Can you work these out from the model? Positions are in its coordinate system, mm. A direction names the side the tool comes from. Give positions to 0.01 mm unless a question says otherwise; leave off trailing zeros. Order: outer loops, then holes, each group sorted by start corner. A loop starts at its lowest first (then second) coordinate and runs counter-clockwise, first axis right, second up. Notation, with made-up numbers: M 19,77.5 L 77,77.5 A17 cw 77,81.5 Z; hole C -37,-37.75 d2. An arc over 180 degrees is marked long. Use one line per item in the form item = value. Start each with the question number.
1. Will these pins go through, and if not, where does the flat tip stop? P1, Ø2, axis at x = -18.5, y = -324, coming from the +Z side; P2, Ø2, axis at x = -17.5, z = -34, coming from the +Y side; P3, Ø2, axis at x = -18, y = -211, coming from the -Z side.
2. I want a section at B-B, the plane x = -2. List the corners of the cut face in (y, z) for me.
3. I need wall thicknesses on L1, parallel to Z at x = 18.85, y = 300; L2, parallel to Z at x = 17.8, y = -103; L3, parallel to Z at x = 2, y = 77.5. Which ranges of each line are inside material? Lowest first, please.
4. I want a section at A-A, the plane y = -191. List the corners of the cut face in (x, z) for me.
5. For faces 4 (the face through (20, 5, -1)), 5 (the face through (16, 5, -1)), which set-ups out of +Z, -Z, +X, -X, +Y, -Y let a thin tool reach every point of the face, with its end or its side?
6. We'd pull the mould along Z, two halves only. Please class faces 1 (the face through (0, 35, -40)), 2 (the face through (-16, 5, 1)), 3 (the face through (0, 4, 40)): +Z half, -Z half, draft (parallel to the pull), parting line (faces both ways), or undercut.
Solid Edge part; units mm, degrees
sketch "Sketch1" plane through (0, 0, 0) normal (0, -1, 0) x (1, 0, 0)
  line L0 (-16, -36) -> (16, -36)
  line L1 (16, -36) -> (16, 36)
  line L2 (16, 36) -> (-16, 36)
  line L3 (-16, 36) -> (-16, -36)
  line L4 (-20, -40) -> (20, -40)
  line L5 (20, -40) -> (20, 40)
  line L6 (20, 40) -> (-20, 40)
  line L7 (-20, 40) -> (-20, -40)
  dimension "D1" = 20
  dimension "D2" = 20
extrude "Protrusion1" add sketch "Sketch1" along normal mid plane 700
sketch "Sketch2" plane through (-20, 0, 0) normal (-1, 0, 0) x (0, -1, 0)
  line L0 (198, -40) -> (218, -40)
  line L1 (218, -40) -> (218, -35)
  line L2 (218, -35) -> (198, -35)
  line L3 (198, -35) -> (198, -40)
  line L4 (-282, -40) -> (-262, -40)
  line L5 (-262, -40) -> (-262, -35)
  line L6 (-262, -35) -> (-282, -35)
  line L7 (-282, -35) -> (-282, -40)
  dimension "D1" = 262
  dimension "D2" = 262
  dimension "D3" = 218
  dimension "D4" = 198
extrude "Cutout1" cut sketch "Sketch2" against normal through all
sketch "Sketch3" plane through (-20, 0, 0) normal (-1, 0, 0) x (0, -1, 0)
  circle A0 centre (-126, 10) radius 3.5
  circle A1 centre (34, 10) radius 3.5
  dimension "D1" = 126
  dimension "D2" = 126
extrude "Cutout2" cut sketch "Sketch3" against normal through all
sketch "Sketch4" plane through (-20, 0, 0) normal (-1, 0, 0) x (0, -1, 0)
  line L0 (350, 40) -> (313.5, 40)
  line L1 (313.5, 40) -> (313.5, 36)
  line L2 (313.5, 36) -> (346, 36)
  line L3 (346, 36) -> (346, 32)
  line L4 (346, 32) -> (350, 32)
  line L5 (350, 32) -> (350, 40)
  dimension "D1" = 350
  dimension "D2" = 313.5
  dimension "D3" = 346
  dimension "D4" = 346
extrude "Cutout3" cut sketch "Sketch4" against normal through all
mirror "Mirror1" about plane through (0, 0, 0) normal (0, 0, 1) of "Cutout3"
mirror "Mirror2" about plane through (0, 0, 0) normal (0, -1, 0) of "Cutout3", "Mirror1"
sketch "Sketch5" plane through (-20, 0, 0) normal (-1, 0, 0) x (0, 1, 0)
  circle A0 centre (-330, 0) radius 3
  circle A1 centre (-300, -25) radius 3
  circle A2 centre (-300, 25) radius 3
  dimension "D1" = 330
extrude "Cutout4" cut sketch "Sketch5" against normal through all
mirror "Mirror3" about plane through (0, 0, 0) normal (0, -1, 0) of "Cutout4"
sketch "Sketch6" plane through (-20, 0, 0) normal (-1, 0, 0) x (0, -1, 0)
  circle A0 centre (241, -27.5) radius 4
  circle A1 centre (241, -9.5) radius 3.25
  circle A2 centre (215, -27.5) radius 3.25
  circle A3 centre (215, -9.5) radius 4
  circle A4 centre (129, -9.5) radius 4
  circle A5 centre (103, -9.5) radius 3.25
  circle A6 centre (103, -27.5) radius 4
  circle A7 centre (129, -27.5) radius 3.25
extrude "Cutout5" cut sketch "Sketch6" against normal through all
properties material "AlSi7Mg"
Check result:
q1.P1 = 36
q1.P2 = 346
q1.P3 = -35
q2.outline = M -313.5,-40 L -218,-40 L -218,-36 L -313.5,-36 Z; M -313.5,36 L 313.5,36 L 313.5,40 L -313.5,40 Z; M -198,-40 L 262,-40 L 262,-36 L -198,-36 Z; M 282,-40 L 313.5,-40 L 313.5,-36 L 282,-36 Z
q3.L1 = -40 to -28, -22 to 22, 28 to 40
q3.L2 = -40 to -31.5, -23.5 to -12.75, -6.25 to 40
q3.L3 = -40 to -36, 36 to 40
q4.outline = M -20,-40 L 20,-40 L 20,40 L -20,40 Z; hole M -16,-36 L 16,-36 L 16,36 L -16,36 Z
q5.face_4 = +Z, -Z, +X, +Y, -Y
q5.face_5 = +Y, -Y
q6.face_1 = -Z half
q6.face_2 = undercut
q6.face_3 = +Z half
